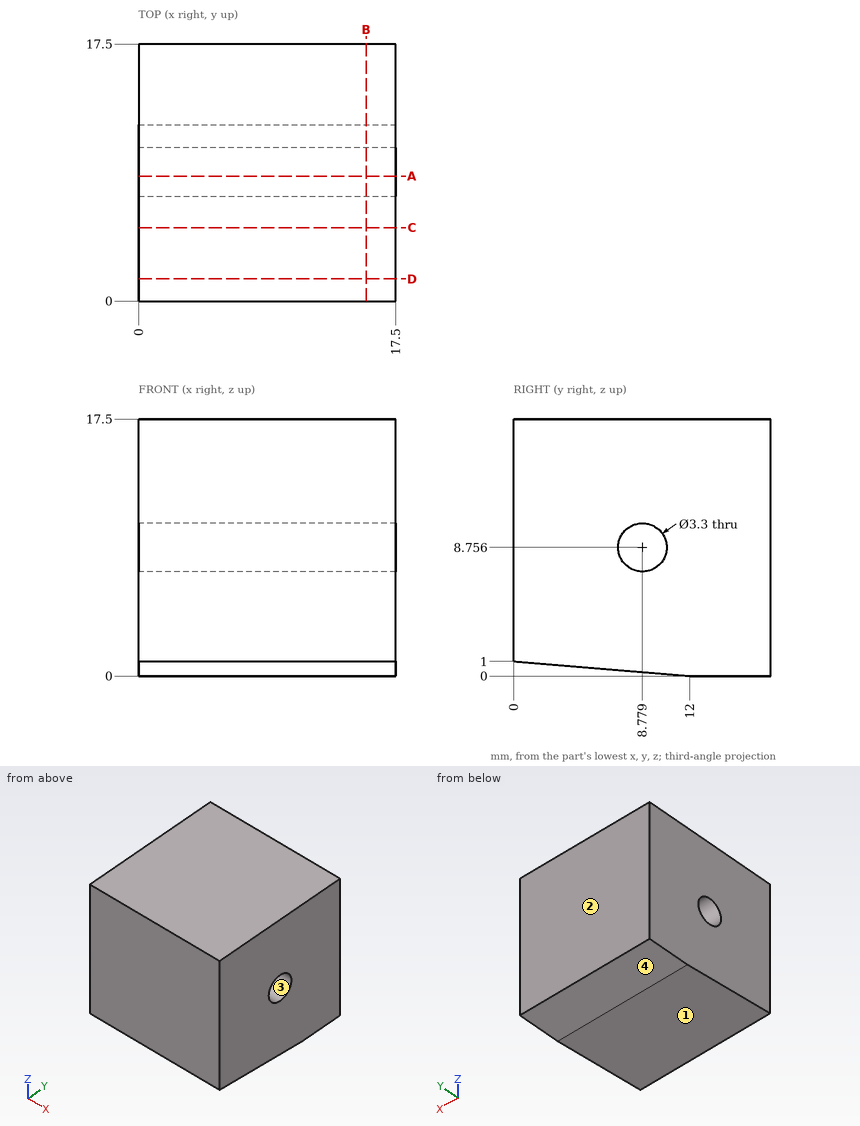
Verification items for this drawing (mm, ordinates from the low corner). Give positions to 0.01 mm unless a question says otherwise; leave off trailing zeros. Loops run counter-clockwise (first coordinate to the right, second up) from the corner with the lowest first, then second, coordinate; pieces in that order, holes last.
1. Material ranges on probe 1 along Z at (x, y) = (5.75, 7.75) (1 decimal); probe 2 along Y at (x, z) = (5.75, 10) (1 decimal); probe 3 along Z at (x, y) = (3, 10) (1 decimal), recorded low to high.
Derived:
probe 1: z = 0.4 to 7.5, 10 to 17.5
probe 2: y = 0 to 7.7, 9.9 to 17.5
probe 3: z = 0.2 to 7.6, 9.9 to 17.5
2. Cross-section at C-C on y = 5. Record the cut outline in (x, z).
Derived:
outline: (0, 0.58) - (17.5, 0.58) - (17.5, 17.5) - (0, 17.5) - close
3. Cross-section at B-B on x = 15.5. Record the cut outline in (y, z).
Derived:
outline: (0, 1) - (12, 0) - (17.5, 0) - (17.5, 17.5) - (0, 17.5) - close; hole circle Ø3.3 at (8.78, 8.76)
4. Go/stop test with a flat-tipped pin: P1, Ø3, axis at y = 8.78, z = 8.76, coming from the -X side. Record where the tip stops, or that it passes through.
Derived:
P1: passes through
5. Cross-section at A-A on y = 8.5. Record the cut outline in (x, z), and give its area (3 significant figures).
Derived:
outline: (0, 0.29) - (17.5, 0.29) - (17.5, 7.13) - (0, 7.13) - close; (0, 10.38) - (17.5, 10.38) - (17.5, 17.5) - (0, 17.5) - close
area: 244 mm2
6. Cross-section at D-D on y = 1.5. Record the cut outline in (x, z) (1 decimal), and give its area (3 significant figures).
Derived:
outline: (0, 0.9) - (17.5, 0.9) - (17.5, 17.5) - (0, 17.5) - close
area: 291 mm2
7. Release check for a two-part mould opening along Y. For the marked faces 1, 2, 3 and 4 record: +Y half, -Y half, draft (parallel to the pull), parting line (faces both ways), or undercut.
Derived:
face 1: -Y half
face 2: +Y half
face 3: undercut
face 4: draft
